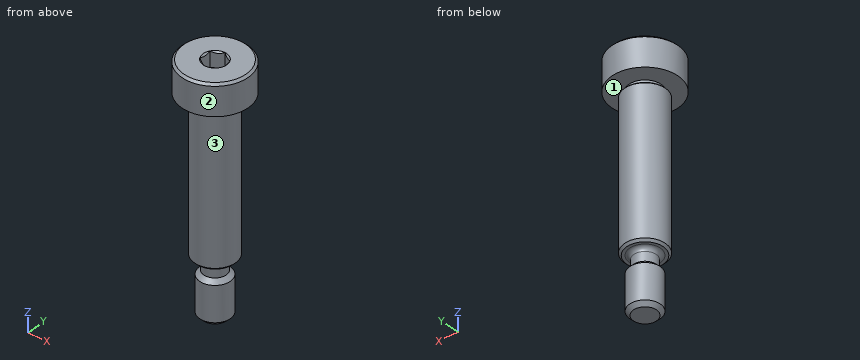
```python
from build123d import *

# Parameters (mm, degrees)
SKETCH4_W          = 0.866666667
SKETCH4_H          = 0.866666667
CHAMFER1_SIZE      = 0.26
CHAMFER2_SIZE      = 0.75
CHAMFER3_SIZE      = 0.4225
CUT_EXTRUDE1_DEPTH = 3


with BuildPart() as part:
    # Sketch3 → Revolve1 (revolve)
    with BuildSketch(Plane(origin=(0, 0, 0), x_dir=(0, 0, -1), z_dir=(1, 0, 0))):
        Polygon((-23.5, 6.5), (-17.5, 6.5), (-17.5, 4), (12.5, 4), (12.5, 3), (23.5, 3), (23.5, 0), (-23.5, 0), align=None)
    revolve(axis=Axis((0, 0, -23.5), (0, 0, 1)))

    # Sketch4 → Cut-Revolve1 (revolve, cut)
    with BuildSketch(Plane(origin=(0, 0, 0), x_dir=(0, 0, -1), z_dir=(1, 0, 0))):
        with Locations((-17.066666666, 3.566666667)):
            Rectangle(SKETCH4_W, SKETCH4_H)
    revolve(axis=Axis((0, 0, -23.5), (0, 0, 1)), mode=Mode.SUBTRACT)

    # Chamfer1
    chamfer1_edges = [part.edges().sort_by_distance(p)[0] for p in [
        (0, -3.133333333, 16.633333333),
        (0, -4, 16.633333333),
    ]]
    chamfer(chamfer1_edges, length=CHAMFER1_SIZE)

    # Sketch6 → Cut-Revolve2 (revolve, cut)
    with BuildSketch(Plane(origin=(0, 0, 0), x_dir=(0, 0, -1), z_dir=(1, 0, 0))):
        with BuildLine():
            Line((12.5, 4), (16.9, 4))
            Line((16.9, 4), (15.1, 2.2))
            Line((15.1, 2.2), (13.3, 2.2))
            ThreePointArc((13.3, 2.2), (12.734314575, 2.434314575), (12.5, 3))
            Line((12.5, 3), (12.5, 4))
        make_face()
    revolve(axis=Axis((0, 0, -23.5), (0, 0, 1)), mode=Mode.SUBTRACT)

    # Chamfer2
    chamfer2_edges = [part.edges().sort_by_distance(p)[0] for p in [
        (0, -3, -23.5),
    ]]
    chamfer(chamfer2_edges, length=CHAMFER2_SIZE)

    # Chamfer3
    chamfer3_edges = [part.edges().sort_by_distance(p)[0] for p in [
        (0, -4, -12.5),
        (0, -6.5, 23.5),
    ]]
    chamfer(chamfer3_edges, length=CHAMFER3_SIZE)

    # Sketch8 → Cut-Extrude1 (cut)
    with BuildSketch(Plane.XY.offset(23.5)):
        Polygon((2, 1.154700538), (0, 2.309401077), (-2, 1.154700538), (-2, -1.154700538), (0, -2.309401077), (2, -1.154700538), align=None)
    extrude(amount=-CUT_EXTRUDE1_DEPTH, mode=Mode.SUBTRACT)

    # Cut-Extrude2 cone 1 section (through the dimple's axis) → Cut-Extrude2 (revolve, cut)
    with BuildSketch(Plane(origin=(0, 0, 23.5), x_dir=(0, -1, 0), z_dir=(1, 0, 0))):
        Polygon((0, 0), (2.309401077, 0), (0, 2.309401077), align=None)
    revolve(axis=Axis((0, 0, 23.5), (0, 0, -1)), mode=Mode.SUBTRACT)


solid = part.part
```
Could you check a few things on this model? Use its own coordinates, in mm. Face numbers are marked on the shaded views. A direction names the side the tool comes from. Give positions to 0.01 mm unless a question says otherwise; leave off trailing zeros. Order: outer loops, then holes, each group sorted by start corner. A loop starts at its lowest first (then second) coordinate and runs counter-clockwise, first axis right, second up.
Q1. If I drill on line 1 along Z through (x, y) = (5, 1.75); line 2 along Z through (x, y) = (-3.5, 0.75); line 3 along Y through (x, z) = (0.25, -3), over which ranges is the centre line in solid material (lowest first)?
Q2. Suppose I cut it at A-A, the plane z = -4. Write out the boundary of the cut face in (x, y), and give its area (3 significant figures).
Q3. I'm going to push flat-ended pins straight in: P1, Ø4.5, axis at x = -0.5, y = 0.5, coming from the +Z side; P2, Ø1, axis at x = 1.5, z = 0.5, coming from the +Y side; P3, Ø1, axis at y = -2.5, z = -2, coming from the +X side; P4, Ø2, axis at x = -3.5, y = 4.5, coming from the -Z side. Where does each tip first touch, or does it pass through?
Q4. For the marked faces 1, 2 and 3, which set-ups out of +Z, -Z, +X, -X, +Y, -Y let a thin tool reach every point of the face, with its end or its side?
Solution:
1. line 1: z = 17.5 to 23.5
1. line 2: z = -12.5 to 16.63, 17.5 to 23.5
1. line 3: y = -3.99 to 3.99
2. outline: circle Ø8 at (0, 0)
2. area: 50.3 mm2
3. P1: stops at z = 23.5
3. P2: stops at y = 3.87
3. P3: stops at x = 3.46
3. P4: stops at z = 17.5
4. face 1: none
4. face 2: +Z, -Z
4. face 3: -Z
